Autodesk Inventor part; units mm, degrees
ref_plane "YZ Plane" through (0, 0, 0) normal (1, 0, 0) x (0, 1, 0)
ref_plane "XZ Plane" through (0, 0, 0) normal (0, 1, 0) x (-1, 0, 0)
ref_plane "XY Plane" through (0, 0, 0) normal (0, 0, 1) x (1, 0, 0)
sketch "Sketch1" plane through (0, 0, 0) normal (0, 0, 1) x (1, 0, 0)
  circle A0 centre (0, 0) radius 19.05
  circle A1 centre (0, 0) radius 15.875 construction
  circle A2 centre (0, 0) radius 11.1125
  line L0 (0, 0) -> (0, 19.05) construction
  circle A3 centre (0, 15.875) radius 1.5
  line L1 (-1.5875, 10.9985) -> (-1.5875, 18.9837)
  line L2 (1.5875, 10.9985) -> (1.5875, 18.9837)
  circle A4 centre (0, 0) radius 7.9375
  arc A5 (-4.6691, 15.1728) -> (-15.1728, 4.6691) centre (0, 0) ccw
  arc A6 (-15.4746, 3.5428) -> (-11.63, -10.8055) centre (0, 0) ccw
  arc A7 (-10.8055, -11.63) -> (3.5428, -15.4746) centre (0, 0) ccw
  arc A8 (4.6691, -15.1728) -> (15.1728, -4.6691) centre (0, 0) ccw
  arc A9 (15.4746, -3.5428) -> (11.63, 10.8055) centre (0, 0) ccw
  arc A10 (10.8055, 11.63) -> (-3.5428, 15.4746) centre (0, 0) ccw
  line L3 (-1.5875, 18.9837) -> (-1.5875, 21.5237) construction
  line L4 (-1.5875, 21.5237) -> (1.5875, 18.9837) construction
  arc A11 (-15.405, -3.8344) -> (-3.8344, -15.405) centre (0, 0) ccw
  arc A12 (4.6691, -15.1728) -> (15.1728, -4.6691) centre (0, 0) ccw
  arc A13 (15.3341, 4.1088) -> (4.6691, 15.1728) centre (0, 0) ccw
  arc A14 (-4.6691, 15.1728) -> (-15.1728, 4.6691) centre (0, 0) ccw
  line L5 (0, 19.05) -> (-2.54, 19.05) construction
  line L6 (-2.54, 19.05) -> (-2.54, 21.5237) construction
  line L7 (-2.54, 21.5237) -> (0, 21.5237) construction
  line L8 (0, 21.5237) -> (0, 19.05) construction
  line L9 (0, 19.05) -> (-2.54, 21.5237)
  line L10 (-2.54, 18.8799) -> (-2.54, 21.5237)
  line L11 (0, 19.05) -> (2.54, 21.5237)
  line L12 (2.54, 18.8799) -> (2.54, 21.5237)
  line L13 (-9.525, 16.4978) -> (-8.5622, 19.9101)
  line L14 (-7.2402, 17.6205) -> (-8.5622, 19.9101)
  line L15 (-9.525, 16.4978) -> (-12.9616, 17.3701)
  line L16 (-11.6397, 15.0805) -> (-12.9616, 17.3701)
  line L17 (-16.4978, 9.525) -> (-17.3701, 12.9616)
  line L18 (-15.0805, 11.6397) -> (-17.3701, 12.9616)
  line L19 (-16.4978, 9.525) -> (-19.9101, 8.5622)
  line L20 (-17.6205, 7.2402) -> (-19.9101, 8.5622)
  line L21 (-19.05, 0) -> (-21.5237, 2.54)
  line L22 (-18.8799, 2.54) -> (-21.5237, 2.54)
  line L23 (-19.05, 0) -> (-21.5237, -2.54)
  line L24 (-18.8799, -2.54) -> (-21.5237, -2.54)
  line L25 (-16.4978, -9.525) -> (-19.9101, -8.5622)
  line L26 (-17.6205, -7.2402) -> (-19.9101, -8.5622)
  line L27 (-16.4978, -9.525) -> (-17.3701, -12.9616)
  line L28 (-15.0805, -11.6397) -> (-17.3701, -12.9616)
  line L29 (-9.525, -16.4978) -> (-12.9616, -17.3701)
  line L30 (-11.6397, -15.0805) -> (-12.9616, -17.3701)
  line L31 (-9.525, -16.4978) -> (-8.5622, -19.9101)
  line L32 (-7.2402, -17.6205) -> (-8.5622, -19.9101)
  line L33 (0, -19.05) -> (-2.54, -21.5237)
  line L34 (-2.54, -18.8799) -> (-2.54, -21.5237)
  line L35 (0, -19.05) -> (2.54, -21.5237)
  line L36 (2.54, -18.8799) -> (2.54, -21.5237)
  line L37 (9.525, -16.4978) -> (8.5622, -19.9101)
  line L38 (7.2402, -17.6205) -> (8.5622, -19.9101)
  line L39 (9.525, -16.4978) -> (12.9616, -17.3701)
  line L40 (11.6397, -15.0805) -> (12.9616, -17.3701)
  line L41 (16.4978, -9.525) -> (17.3701, -12.9616)
  line L42 (15.0805, -11.6397) -> (17.3701, -12.9616)
  line L43 (16.4978, -9.525) -> (19.9101, -8.5622)
  line L44 (17.6205, -7.2402) -> (19.9101, -8.5622)
  line L45 (19.05, 0) -> (21.5237, -2.54)
  line L46 (18.8799, -2.54) -> (21.5237, -2.54)
  line L47 (19.05, 0) -> (21.5237, 2.54)
  line L48 (18.8799, 2.54) -> (21.5237, 2.54)
  line L49 (16.4978, 9.525) -> (19.9101, 8.5622)
  line L50 (17.6205, 7.2402) -> (19.9101, 8.5622)
  line L51 (16.4978, 9.525) -> (17.3701, 12.9616)
  line L52 (15.0805, 11.6397) -> (17.3701, 12.9616)
  line L53 (9.525, 16.4978) -> (12.9616, 17.3701)
  line L54 (11.6397, 15.0805) -> (12.9616, 17.3701)
  line L55 (9.525, 16.4978) -> (8.5622, 19.9101)
  line L56 (7.2402, 17.6205) -> (8.5622, 19.9101)
  arc A15 (4.6691, 15.1728) -> (3.2684, 10.621) centre (3.9687, 12.8969) ccw
  arc A16 (-3.2684, 10.621) -> (-4.6691, 15.1728) centre (-3.9687, 12.8969) ccw
  arc A17 (-15.1728, 4.6691) -> (-10.621, 3.2684) centre (-12.8969, 3.9688) ccw
  line L57 (-10.9985, 1.5875) -> (-18.9837, 1.5875)
  circle A18 centre (-15.875, 0) radius 1.5
  line L58 (-10.9985, -1.5875) -> (-18.9837, -1.5875)
  arc A19 (-10.621, -3.2684) -> (-15.1728, -4.6691) centre (-12.8969, -3.9688) ccw
  arc A20 (-4.6691, -15.1728) -> (-3.2684, -10.621) centre (-3.9688, -12.8969) ccw
  line L59 (-1.5875, -10.9985) -> (-1.5875, -18.9837)
  circle A21 centre (0, -15.875) radius 1.5
  line L60 (1.5875, -10.9985) -> (1.5875, -18.9837)
  arc A22 (3.2684, -10.621) -> (4.6691, -15.1728) centre (3.9687, -12.8969) ccw
  arc A23 (15.1728, -4.6691) -> (10.621, -3.2684) centre (12.8969, -3.9688) ccw
  line L61 (10.9985, -1.5875) -> (18.9837, -1.5875)
  circle A24 centre (15.875, 0) radius 1.5
  line L62 (10.9985, 1.5875) -> (18.9837, 1.5875)
  arc A25 (10.621, 3.2684) -> (15.1728, 4.6691) centre (12.8969, 3.9688) ccw
  point P0 (1.5875, 14.665)
  point P1 (4.5184, 10.1524)
  point P2 (10.8055, 11.63)
  point P3 (11.63, 10.8055)
  point P4 (-10.8055, -11.63)
  point P5 (-11.63, -10.8055)
  point P6 (-11.6397, 15.0805)
  point P7 (-9.525, 16.4978)
  point P8 (-9.525, 16.4978)
  point P9 (-7.2402, 17.6205)
  point P10 (-17.6205, 7.2402)
  point P11 (-16.4978, 9.525)
  point P12 (-16.4978, 9.525)
  point P13 (-15.0805, 11.6397)
  point P14 (-18.8799, -2.54)
  point P15 (-19.05, 0)
  point P16 (-19.05, 0)
  point P17 (-18.8799, 2.54)
  point P18 (-15.0805, -11.6397)
  point P19 (-16.4978, -9.525)
  point P20 (-16.4978, -9.525)
  point P21 (-17.6205, -7.2402)
  point P22 (-7.2402, -17.6205)
  point P23 (-9.525, -16.4978)
  point P24 (-9.525, -16.4978)
  point P25 (-11.6397, -15.0805)
  point P26 (2.54, -18.8799)
  point P27 (0, -19.05)
  point P28 (0, -19.05)
  point P29 (-2.54, -18.8799)
  point P30 (11.6397, -15.0805)
  point P31 (9.525, -16.4978)
  point P32 (9.525, -16.4978)
  point P33 (7.2402, -17.6205)
  point P34 (17.6205, -7.2402)
  point P35 (16.4978, -9.525)
  point P36 (16.4978, -9.525)
  point P37 (15.0805, -11.6397)
  point P38 (19.05, 0)
  point P39 (19.05, 0)
  point P40 (18.8799, -2.54)
  point P41 (18.8799, 2.54)
  point P42 (15.0805, 11.6397)
  point P43 (16.4978, 9.525)
  point P44 (16.4978, 9.525)
  point P45 (17.6205, 7.2402)
  point P46 (7.2402, 17.6205)
  point P47 (9.525, 16.4978)
  point P48 (9.525, 16.4978)
  point P49 (11.6397, 15.0805)
  point P50 (-14.665, 1.5875)
  point P51 (-1.5875, -14.665)
  point P52 (14.665, -1.5875)
  point P53 (3.2684, -10.621)
  point P54 (10.621, -3.2684)
  point P55 (15.1728, -4.6691)
  point P56 (4.6691, -15.1728)
  point P57 (-3.2684, -10.621)
  point P58 (-4.6691, -15.1728)
  point P59 (-15.1728, -4.6691)
  point P60 (-3.2684, 10.621)
  point P61 (-10.621, 3.2684)
  point P62 (-15.1728, 4.6691)
  point P63 (4.6691, 15.1728)
  point P64 (15.1728, 4.6691)
  point P65 (10.621, 3.2684)
  dimension "d0" = 38.1
  dimension "d1" = 31.75
  dimension "d2" = 22.225
  dimension "d3" = 3
  dimension "d4" = 1.5875
  dimension "d5" = 1.5875
  dimension "d10" = 15.875
  dimension "d13" = 360
  dimension "d15" = 2.54
  dimension "d22" = 2.54
  dimension "d25" = 360
  dimension "d29" = 360
extrude "Extrusion1" add sketch "Sketch1" along normal blind 1 contours A0 L61 A9 A24 L62 | L45 L46 A0 | A0 L48 L47 | L62 A9 A13 A10 L2 A0 | A0 L60 A22 A8 A23 L61 | L62 A25 A9 | A9 A24 L61 A2 L62 | A0 L49 L50 | L62 A2 A25 | L44 L43 A0 | A23 A2 L61 | A0 L52 L51 | A2 | L41 L42 A0 | A2 L2 A15 | A22 L60 A2 | A0 L53 L54 | A2 L1 A10 A3 L2 | L2 A10 A15 | L40 L39 A0 | L60 A7 A21 L59 A2 | A0 L56 L55 | A2 A16 L1 | A10 A3 L1 A0 L2 | L37 L38 A0 | L60 A0 L59 A7 A21 | L59 A20 A2 | A16 A5 A17 L57 A0 L1 | A0 L11 L12 | A0 L36 L35 | L59 A7 A20 | A2 L57 A17 | A0 L10 L9 | L33 L34 A0 | A19 L58 A2 | A7 L59 A0 L58 A6 A11 | A2 L58 A6 A18 L57 | A19 A6 L58 | A6 A18 L58 A0 L57 | A0 L21 L22 | A0 L13 L14 | L32 L31 A0 | A0 L24 L23 | A0 L16 L15 | L29 L30 A0 | L20 L19 A0 | A0 L25 L26 | L17 L18 A0 | L28 L27 A0
equation "\"OD\" = 38.1"
properties part number "Wood Magnets  (UNI) V1.0." material "Titanium"
CAD build for the part. Positions are in the model's coordinates, mm. A direction names the side the tool comes from. Coordinates: 2 decimals unless noted, no trailing zeros. Write each loop counter-clockwise with the first axis right and the second up, starting at its lowest first coordinate (ties: lowest second). Pieces come first, ordered by that corner, then holes. Notation, with made-up numbers: M 52.25,-31 L 88.25,-31 A24 ccw 88.25,-18 Z; hole C -23,17 d8. An arc over 180 degrees is marked long. Answer as a JSON object with one key per item and string values. Group by question number.
1) Pin check, flat tips, straight feed: pin 1 Ø0.5 at (x, z) = (20.5, 0.5) entering from -Y; pin 2 Ø2.5 at (x, y) = (15.875, 0) entering from -Z; pin 3 Ø0.5 at (y, z) = (20.5, 0.5) entering from -X; pin 4 Ø0.5 at (x, z) = (20, 0.5) entering from +Y. Stop position of each tip, or through.
2) Saw through at B-B (y = -4). Write the cut outline in (x, z), plus the area to 3 significant figures.
3) Tool access for faces 5 (the face through (2.54, -20.2, 0.5)), 6 (the face through (-13.49, 13.45, 0.49)), 7 (the face through (-20.2, -2.54, 0.5)): list every direction of +Z, -Z, +X, -X, +Y, -Y with a clear straight run to the whole face (end or side of a thin tool).
4) Saw through at C-C (z = 0.2). Give the number of separate pieces and of enclosed holes in the cut face, plus the area to 3 significant figures.
5) Mould opens along X. For faces 1 (the face through (-20.27, 1.25, 0.49)), 2 (the face through (4.9, 18.41, 0.49)), 3 (the face through (18.749, -7.892, 0.493)), 4 (the face through (20.2, 2.54, 0.5)) say: +X half, -X half, draft (parallel to the pull), parting line (faces both ways), or undercut.
6) Wall check: line 1 (Y direction, x = -10, z = 0.6); line 2 (X direction, y = 3, z = 0.9); line 3 (X direction, y = -1, z = 0.85). Give the ranges that are in metal, low to high. Write a range as from..to.
7) Saw through at A-A (x = -6). Write the cut outline in (y, z).
Values follow:
{
 "1": {"pin 1": "stops at y = -2.54", "pin 2": "passes through", "pin 3": "stops at x = -2.54", "pin 4": "stops at y = 8.61"},
 "2": {"outline": "M -18.63,0 L -15.28,0 L -15.28,1 L -18.63,1 Z; M -10.37,0 L -6.86,0 L -6.86,1 L -10.37,1 Z; M 6.86,0 L 10.37,0 L 10.37,1 L 6.86,1 Z; M 15.28,0 L 18.63,0 L 18.63,1 L 15.28,1 Z", "area": "13.7 mm2"},
 "3": {"face 5": "+Z, -Z, -Y", "face 6": "+Z, -Z", "face 7": "+Z, -Z, -X"},
 "4": {"separate pieces": "1", "enclosed holes": "9", "area": "671 mm2"},
 "5": {"face 1": "-X half", "face 2": "undercut", "face 3": "+X half", "face 4": "draft"},
 "6": {"line 1": "y = -16.62..-12.33, -4.85..4.85, 12.33..16.62", "line 2": "x = -18.81..-15.07, -10.72..-7.35, 7.35..10.72, 15.07..18.81", "line 3": "x = -20.02..-16.99, -14.76..-7.87, 7.87..14.76, 16.99..20.02"},
 "7": {"outline": "M -18.08,0 L -14.7,0 L -14.7,1 L -18.08,1 Z; M -9.35,0 L -5.2,0 L -5.2,1 L -9.35,1 Z; M 5.2,0 L 9.35,0 L 9.35,1 L 5.2,1 Z; M 14.7,0 L 18.08,0 L 18.08,1 L 14.7,1 Z"}
}
